The model under review builds one solid part; all positions refer to its coordinate system, in mm. Face numbers are marked on the shaded views. A direction names the side the tool comes from. Give positions to 0.01 mm unless a question says otherwise; leave off trailing zeros. Write each loop counter-clockwise with the first axis right and the second up, starting at its lowest first coordinate (ties: lowest second). Pieces come first, ordered by that corner, then holes. Notation, with made-up numbers: (-38.5, -4) - (-11.5, -4) arc R17 cw to (-11.5, 25) - close; hole circle Ø5 at (72.5, 5.5). An arc over 180 degrees is marked (long way). One line per question, with ' | ' between items. Start each with the question number.
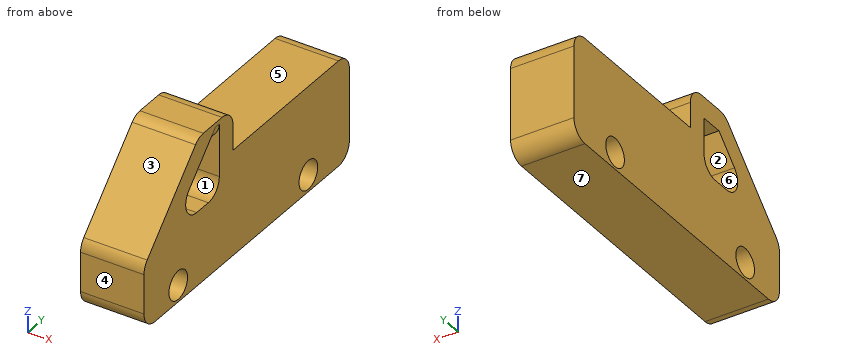
```python
from build123d import *

# Parameters (mm, degrees)
F0_R     = 6.7962511827
F1_DEPTH = 15
F2_R     = 8


with BuildPart() as f1:
    # F0 (on Right) → F1 (new body, symmetric)
    with BuildSketch(Plane.YZ):
        Polygon((0, 30), (0, 0), (150, 0), (150, 50), (65, 50), (65, 70), (40, 70), align=None)
        with Locations((25, 8)):
            Circle(F0_R, mode=Mode.SUBTRACT)
        with Locations((120, 8)):
            Circle(F0_R, mode=Mode.SUBTRACT)
        Polygon((44.1421356237, 60), (55, 60), (55, 35), (19.1421356237, 35), align=None, mode=Mode.SUBTRACT)
    extrude(amount=F1_DEPTH, both=True)

    # F2 (call 1 of 9: OpenCascade refuses the feature's edges together)
    f2_edges = [f1.edges().sort_by_distance(p)[0] for p in [
        (0, 40, 70),
    ]]
    fillet(f2_edges, radius=F2_R)

    # F2#2 (call 2 of 9)
    f2_2_edges = [f1.edges().sort_by_distance(p)[0] for p in [
        (0, 65, 70),
    ]]
    fillet(f2_2_edges, radius=F2_R)

    # F2#3 (call 3 of 9)
    f2_3_edges = [f1.edges().sort_by_distance(p)[0] for p in [
        (0, 150, 50),
    ]]
    fillet(f2_3_edges, radius=F2_R)

    # F2#4 (call 4 of 9)
    f2_4_edges = [f1.edges().sort_by_distance(p)[0] for p in [
        (0, 0, 30),
    ]]
    fillet(f2_4_edges, radius=F2_R)

    # F2#5 (call 5 of 9)
    f2_5_edges = [f1.edges().sort_by_distance(p)[0] for p in [
        (0, 0, 0),
    ]]
    fillet(f2_5_edges, radius=F2_R)

    # F2#6 (call 6 of 9)
    f2_6_edges = [f1.edges().sort_by_distance(p)[0] for p in [
        (0, 150, 0),
    ]]
    fillet(f2_6_edges, radius=F2_R)

    # F2#7 (call 7 of 9)
    f2_7_edges = [f1.edges().sort_by_distance(p)[0] for p in [
        (0, 19.142136, 35),
    ]]
    fillet(f2_7_edges, radius=F2_R)

    # F2#8 (call 8 of 9)
    f2_8_edges = [f1.edges().sort_by_distance(p)[0] for p in [
        (15, 49.571068, 60),
    ]]
    fillet(f2_8_edges, radius=F2_R)

    # F2#9 (call 9 of 9)
    f2_9_edges = [f1.edges().sort_by_distance(p)[0] for p in [
        (0, 55, 35),
    ]]
    fillet(f2_9_edges, radius=F2_R)


solid = f1.part
```
Item 1: Take a section at B-B (y = 120). Give the boundary of the cut face in (x, z).
Item 2: Take a section at D-D (y = 85.5). Give the boundary of the cut face in (x, z), plus the area to 3 significant figures.
Item 3: Take a section at C-C (z = 39.5). Give the boundary of the cut face in (x, y).
Item 4: For probe 1 along Z at (x, y) = (6.75, 120); probe 2 along Z at (x, y) = (-7.25, 66.5); probe 3 along Y at (x, z) = (13.25, 10), list the stretches that pass through material, from the lowest coordinate up.
Item 5: Clearance check with flat-ended pins moving along their axes: P1, Ø1, axis at x = -4, z = 46.5, coming from the -Y side; P2, Ø4.5, axis at x = 1.5, y = 42.5, coming from the +Z side; P3, Ø4, axis at x = 6, y = 97.5, coming from the +Z side; P4, Ø6, axis at x = -2.5, z = 54.5, coming from the +Y side. State where each tip first meets the part, or that it passes through.
Item 6: Take a section at A-A (x = 3). Give the boundary of the cut face in (y, z), plus the area to 3 significant figures.
Item 7: Machinability: for the marked faces 5, 6 and 7, which of the approach directions +Z, -Z, +X, -X, +Y, -Y give a long, thin tool a straight path to every point of the face, cutting with its end or side? Answer none if there is none.
Item 8: The part is to be moulded in two halves that separate along Z. For the marked faces 1, 2, 3 and 4, say which applies: +Z half, -Z half, draft (parallel to the pull), parting line (faces both ways), or undercut.
Check sheet entries:
1) outline: (-15, 0) - (15, 0) - (15, 1.2) - (-15, 1.2) - close; (-15, 14.8) - (15, 14.8) - (15, 50) - (-15, 50) - close
2) outline: (-15, 0) - (15, 0) - (15, 50) - (-15, 50) - close | area: 1,500 mm^2
3) outline: (-15, 9.5) - (15, 9.5) - (15, 31.26) - (-15, 31.26) - close; (-15, 54.19) - (15, 54.19) - (15, 150) - (-15, 150) - close
4) probe 1: z = 0 to 1.2, 14.8 to 50 | probe 2: z = 0 to 50 | probe 3: y = 0 to 18.5, 31.5 to 113.5, 126.5 to 150
5) P1: stops at y = 16 | P2: stops at z = 70 | P3: stops at z = 50 | P4: stops at y = 65
6) outline: (0, 8) arc R8 ccw to (8, 0) - (142, 0) arc R8 ccw to (150, 8) - (150, 42) arc R8 ccw to (142, 50) - (65, 50) - (65, 62) arc R8 ccw to (57, 70) - (43.31, 70) arc R8 ccw to (37.66, 67.66) - (2.34, 32.34) arc R8 ccw to (0, 26.69) - close; hole circle Ø13.59 at (25, 8); hole (32.8, 48.66) arc R8 ccw to (38.46, 35) - (47, 35) arc R8 ccw to (55, 43) - (55, 60) - (44.14, 60) - close; hole circle Ø13.59 at (120, 8) | area: 7,160 mm^2
7) face 5: +Z, +X, -X, +Y | face 6: +X, -X | face 7: -Z, +X, -X, +Y, -Y
8) face 1: undercut | face 2: undercut | face 3: +Z half | face 4: draft
